Verification items for the finished model (mm, model axes). Face numbers are marked on the shaded views. A direction names the side the tool comes from. Round coordinates to 2 decimals unless told otherwise and drop trailing zeros. Order: outer loops, then holes, each group sorted by start corner. A loop starts at its lowest first (then second) coordinate and runs counter-clockwise, first axis right, second up. Notation, with made-up numbers: M 46,68.25 L 80,68.25 A24 ccw 80,84.25 Z; hole C -12,59.5 d8. An arc over 180 degrees is marked long. Answer as a JSON object with one key per item and string values. Group by question number.
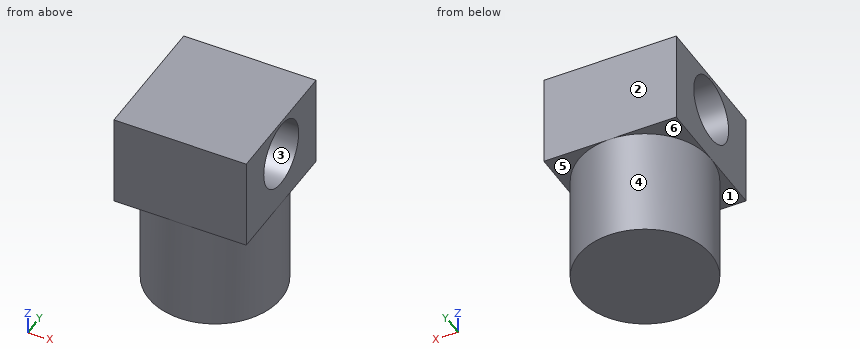
```python
from build123d import *

# Parameters (mm, degrees)
F0_R     = 100
F1_DEPTH = 265
F2_R     = 100
F3_DEPTH = 100
F4_W     = 200
F4_H     = 200
F5_DEPTH = 140
F6_R     = 50
F7_DEPTH = 200


with BuildPart() as f1:
    # F0 (on Top) → F1 (new body)
    with BuildSketch(Plane.XY):
        Circle(F0_R)
    extrude(amount=F1_DEPTH)

    # F2 (on face) → F3 (cut)
    with BuildSketch(Plane(origin=(0, 0, 0), x_dir=(1, 0, 0), z_dir=(0, 0, -1))):
        Circle(F2_R)
    extrude(amount=-F3_DEPTH, mode=Mode.SUBTRACT)

    # F4 (on face) → F5 (join)
    with BuildSketch(Plane.XY.offset(265)):
        Rectangle(F4_W, F4_H)
    extrude(amount=F5_DEPTH)

    # F6 (on face) → F7 (cut)
    with BuildSketch(Plane(origin=(-100, 0, 0), x_dir=(0, -1, 0), z_dir=(-1, 0, 0))):
        with Locations((0, 350)):
            Circle(F6_R)
    extrude(amount=-F7_DEPTH, mode=Mode.SUBTRACT)


solid = f1.part
```
Q1. Gauge pin test, flat ends, axial feed: pin 1 Ø3 at (y, z) = (-74, 230) entering from -X; pin 2 Ø10 at (y, z) = (-16.5, 231) entering from -X; pin 3 Ø4 at (x, z) = (47, 227.5) entering from +Y. Record the tip position at first contact, or that the pin passes through.
Q2. Thickness scan on line 1 (Z direction, x = -34, y = 0); line 2 (Z direction, x = 66, y = 32.5); line 3 (Y direction, x = -68, z = 371). Record the ranges inside material, lowest first. Write a range as from..to.
Q3. Cross-section at B-B, the plane y = 15. Record the cut outline in (x, z).
Q4. Cross-section at C-C, the plane x = 5.5. Record the cut outline in (y, z), then the cut area to 3 significant figures.
Q5. Cross-section at A-A, the plane z = 350. Record the cut outline in (x, y).
Q6. Release check for a two-part mould opening along Z. For the marked faces 1, 2 and 3 record: released by +Z, released by -Z, zero draft, split by the parting line, or undercut.
Q7. Cross-section at D-D, the plane y = 61. Record the cut outline in (x, z), then the cut area to 3 significant figures.
Q8. Tool access check on the marked faces 4, 5 and 6. Record the directions out of +Z, -Z, +X, -X, +Y, -Y that give a thin tool (end or side, any length) a straight path to the whole face; none if there is none.
Conclusion:
{
 "1": {"pin 1": "x = -68.87", "pin 2": "x = -99.34", "pin 3": "y = 89.3"},
 "2": {"line 1": "100..300, 400..405", "line 2": "100..312, 388..405", "line 3": "-100..-45.38, 45.38..100"},
 "3": {"outline": "M -100,265 L -98.87,265 L -98.87,100 L 98.87,100 L 98.87,265 L 100,265 L 100,302.3 L -100,302.3 Z; M -100,397.7 L 100,397.7 L 100,405 L -100,405 Z"},
 "4": {"outline": "M -100,265 L -99.85,265 L -99.85,100 L 99.85,100 L 99.85,265 L 100,265 L 100,405 L -100,405 Z; hole C 0,350 d100", "area": "53,100 mm2"},
 "5": {"outline": "M -100,-100 L 100,-100 L 100,-50 L -100,-50 Z; M -100,50 L 100,50 L 100,100 L -100,100 Z"},
 "6": {"face 1": "released by -Z", "face 2": "zero draft", "face 3": "undercut"},
 "7": {"outline": "M -100,265 L -79.24,265 L -79.24,100 L 79.24,100 L 79.24,265 L 100,265 L 100,405 L -100,405 Z", "area": "54,100 mm2"},
 "8": {"face 4": "-Z", "face 5": "-Z, +X, +Y", "face 6": "-Z, -X, +Y"}
}
